Read the model definition and answer for the solid it produces. Units are mm, in the model's axes. A direction names the side the tool comes from. Coordinates: 2 decimals unless noted, no trailing zeros. Write each loop counter-clockwise with the first axis right and the second up, starting at its lowest first coordinate (ties: lowest second). Pieces come first, ordered by that corner, then holes. Notation, with made-up numbers: (58.5, -33.5) -> (85.5, -33.5) arc R32 cw to (85.5, -0.5) -> close; hole circle Ø10 at (30, 79). An arc over 180 degrees is marked (long way). Return JSON: item names as keys, results as strings.
from build123d import *

# Parameters (mm, degrees)
BOSS_EXTRUDE1_DEPTH = 4


with BuildPart() as part:
    # Sketch1 → Boss-Extrude1 (new body)
    with BuildSketch(Plane(origin=(0, 0, 0), x_dir=(1, 0, 0), z_dir=(0, 1, 0))):
        with BuildLine():
            ThreePointArc((30.815272538, -36.001699489), (25.402435992, -38.396198014), (19.625399795, -39.683938449))
            ThreePointArc((19.625399795, -39.683938449), (11.702107234, -40.100543502), (3.79576222, -39.435838094))
            Line((3.79576222, -39.435838094), (3.644269307, -40.424296438))
            ThreePointArc((3.644269307, -40.424296438), (11.686436005, -41.100420701), (19.745841387, -40.676658864))
            ThreePointArc((19.745841387, -40.676658864), (25.715015737, -39.346089535), (31.307877538, -36.871952506))
            Line((31.307877538, -36.871952506), (39.401230599, -32.290726007))
            ThreePointArc((39.401230599, -32.290726007), (40.654759367, -31.420634412), (41.728618671, -30.336558791))
            Line((41.728618671, -30.336558791), (46.115294675, -25.01048391))
            ThreePointArc((46.115294675, -25.01048391), (46.926204525, -23.750298002), (47.422252359, -22.336232991))
            Line((47.422252359, -22.336232991), (48.929279873, -15.602818696))
            ThreePointArc((48.929279873, -15.602818696), (49.083336252, -14.112211456), (48.886975652, -12.626585049))
            Line((48.886975652, -12.626585049), (47.189177971, -5.938724177))
            ThreePointArc((47.189177971, -5.938724177), (46.653139583, -4.539329252), (45.806739977, -3.302700361))
            Line((45.806739977, -3.302700361), (41.270456965, 1.896543473))
            ThreePointArc((41.270456965, 1.896543473), (40.159986728, 2.902773645), (38.846178779, 3.62357319))
            Line((38.846178779, 3.62357319), (28.678343339, 7.739009747))
            ThreePointArc((28.678343339, 7.739009747), (26.957465579, 8.469564765), (25.262216259, 9.257765654))
            ThreePointArc((25.262216259, 9.257765654), (23.267121819, 9.961406596), (21.165078625, 10.2))
            Line((21.165078625, 10.2), (0, 10.2))
            ThreePointArc((0, 10.2), (-2.249376643, 9.649581037), (-3.9904429, 8.122706909))
            Line((-3.9904429, 8.122706909), (-15.810441253, -8.758000179))
            ThreePointArc((-15.810441253, -8.758000179), (-17.037346005, -12.320539523), (-16.190374911, -15.991999971))
            Line((-16.190374911, -15.991999971), (-5.517086169, -35.257340666))
            ThreePointArc((-5.517086169, -35.257340666), (-4.183080077, -36.586813335), (-2.345658451, -37.000276272))
            ThreePointArc((-2.345658451, -37.000276272), (0.184189718, -37.023630883), (2.686718995, -37.395147249))
            ThreePointArc((2.686718995, -37.395147249), (2.95899063, -37.449951511), (3.233042455, -37.495017541))
            ThreePointArc((3.233042455, -37.495017541), (17.592116724, -37.228639758), (31.102694288, -32.358499632))
            Line((31.102694288, -32.358499632), (30.614795368, -31.485599499))
            ThreePointArc((30.614795368, -31.485599499), (17.410864376, -36.245203137), (3.377694822, -36.505535003))
            ThreePointArc((3.377694822, -36.505535003), (3.138815013, -36.466252781), (2.901486924, -36.418482139))
            ThreePointArc((2.901486924, -36.418482139), (0.262415361, -36.026695204), (-2.405465658, -36.002066325))
            ThreePointArc((-2.405465658, -36.002066325), (-3.701447688, -35.710439989), (-4.642357438, -34.772727782))
            Line((-4.642357438, -34.772727782), (-15.31564618, -15.507387087))
            ThreePointArc((-15.31564618, -15.507387087), (-16.038722362, -12.372987788), (-14.991289209, -9.331576615))
            Line((-14.991289209, -9.331576615), (-3.171290856, 7.549130473))
            ThreePointArc((-3.171290856, 7.549130473), (-1.78762803, 8.762570204), (0, 9.2))
            Line((0, 9.2), (21.174669732, 9.2))
            ThreePointArc((21.174669732, 9.2), (22.380727426, 9.083680421), (23.542324402, 8.739009747))
            Line((23.542324402, 8.739009747), (32.075036736, 5.285390097))
            Line((32.075036736, 5.285390097), (38.470995099, 2.696622703))
            ThreePointArc((38.470995099, 2.696622703), (39.579771769, 2.088310262), (40.516943366, 1.239111152))
            Line((40.516943366, 1.239111152), (45.053226377, -3.960132681))
            ThreePointArc((45.053226377, -3.960132681), (45.767537886, -5.003774765), (46.219922772, -6.184781812))
            Line((46.219922772, -6.184781812), (47.917720454, -12.872642684))
            ThreePointArc((47.917720454, -12.872642684), (48.083437256, -14.126424033), (47.953422729, -15.384408911))
            Line((47.953422729, -15.384408911), (46.446395215, -22.117823206))
            ThreePointArc((46.446395215, -22.117823206), (46.027760006, -23.311210944), (45.343399765, -24.374733765))
            Line((45.343399765, -24.374733765), (40.956723761, -29.700808646))
            ThreePointArc((40.956723761, -29.700808646), (40.011729115, -30.654793636), (38.908625599, -31.42047299))
            Line((38.908625599, -31.42047299), (30.815272538, -36.001699489))
        make_face()
    extrude(amount=BOSS_EXTRUDE1_DEPTH)


solid = part.part
1. The part is cut by section A-A (x = 5). Determine the outline of the cut face in (y, z).
Taken from the geometry:
{"outline": "(0, -10.2) -> (4, -10.2) -> (4, -9.2) -> (0, -9.2) -> close; (0, 36.71) -> (4, 36.71) -> (4, 37.72) -> (0, 37.72) -> close; (0, 39.61) -> (4, 39.61) -> (4, 40.62) -> (0, 40.62) -> close"}
2. For a pull along Z with two mould halves and no side action, classify faces 3 (the face through (26.98, 1.97, -8.46)), 4 (the face through (-10.93, 1.97, 25.49)), 5 (the face through (46.036, 1.972, 23.295)) as +Z half, -Z half, draft (parallel to the pull), parting line (faces both ways), or undercut.
Taken from the geometry:
{"face 3": "-Z half", "face 4": "+Z half", "face 5": "undercut"}
3. Consider L1, parallel to Z at x = 20, y = 2.5; L2, parallel to Z at x = 17.5, y = 3.1; L3, parallel to Z at x = 34.5, y = 3.2. Determine where each line is inside the solid, lowest interval first.
Taken from the geometry:
{"L1": "z = -10.2 to -9.2, 35.69 to 36.71, 39.64 to 40.64", "L2": "z = -10.2 to -9.2, 36.23 to 37.25, 39.9 to 40.91", "L3": "z = -5.38 to -4.3, 33.92 to 35.07"}
4. A tool of negligible diameter and unlimited length cuts with its end or side. For faces 1 (the face through (48.165, 1.972, 19.017)), 2 (the face through (45.76, 1.97, 4.99)), from which of +Z, -Z, +X, -X, +Y, -Y can it reach the whole face along a straight path? Write none if from no direction.
Taken from the geometry:
{"face 1": "+Z, +X, +Y, -Y", "face 2": "+Y, -Y"}
5. The part is cut by section C-C (x = 34.5). Determine the outline of the cut face in (y, z), then the cut area to 3 significant figures.
Taken from the geometry:
{"outline": "(0, -5.38) -> (4, -5.38) -> (4, -4.3) -> (0, -4.3) -> close; (0, 33.92) -> (4, 33.92) -> (4, 35.07) -> (0, 35.07) -> close", "area": "8.91 mm2"}
6. Flat-ended cylindrical pins translate along their axes: pin 1 Ø1.5 at (x, y) = (2, 3.5) entering from +Z; pin 2 Ø1 at (x, y) = (5.5, 2.5) entering from +Z; pin 3 Ø1 at (y, z) = (3.5, 1.5) entering from +X. Find the tip coordinate at first contact, or state that the pin passes through.
Taken from the geometry:
{"pin 1": "stops at z = 37.41", "pin 2": "stops at z = 40.74", "pin 3": "stops at x = 44.67"}
7. The part is cut by section B-B (z = 1.5). Determine the outline of the cut face in (x, y).
Taken from the geometry:
{"outline": "(-10.73, 0) -> (-9.51, 0) -> (-9.51, 4) -> (-10.73, 4) -> close; (42.91, 0) -> (44.23, 0) -> (44.23, 4) -> (42.91, 4) -> close"}
8. The part is cut by section D-D (x = 22). Determine the outline of the cut face in (y, z).
Taken from the geometry:
{"outline": "(0, -10.16) -> (4, -10.16) -> (4, -9.15) -> (0, -9.15) -> close; (0, 35.14) -> (4, 35.14) -> (4, 36.18) -> (0, 36.18) -> close; (0, 39.3) -> (4, 39.3) -> (4, 40.32) -> (0, 40.32) -> close"}
